Geometry check sheet. Reference: the model listing, model coordinates, mm. Face numbers are marked on the shaded views. A direction names the side the tool comes from. Round coordinates to 2 decimals unless told otherwise and drop trailing zeros. Loops run counter-clockwise (first coordinate to the right, second up) from the corner with the lowest first, then second, coordinate; pieces in that order, holes last. Notation, with made-up numbers: (-39, 15) - (-14, 15) arc R4 cw to (-14, 20) - close; hole circle Ø3 at (64.25, 14). An arc over 180 degrees is marked (long way). Answer as CSV lines item,"result". Start each with the question number.
1) Cross-section at A-A on y = 0. Record the boundary of the cut face in (x, z).
2) Thickness scan on line 1 along Y through (x, z) = (0, -2.15); line 2 along Z through (x, y) = (12.5, -9.5); line 3 along Z through (x, y) = (11, 13). Record the ranges inside material, lowest first.
3) Cross-section at B-B on z = -32.5. Record the boundary of the cut face in (x, y), and give its area (3 significant figures).
4) Cross-section at D-D on y = 4. Record the boundary of the cut face in (x, z).
5) Depth check by flat-ended pin: P1, Ø1.5, axis at x = -3.5, z = -52.5, coming from the -Y side; P2, Ø4, axis at x = 0, y = 15.5, coming from the +Z side; P3, Ø1, axis at y = -14.5, z = -46.5, coming from the -X side; P4, Ø11, axis at x = 2.5, y = -4.5, coming from the +Z side. Enter the tip coordinate at first touch or a pass-through.
6) Access from +Z, -Z, +X, -X, +Y, -Y to the whole of each face (thin tool, end or side, straight path). Record for the marked faces 1, 2 and 3.
7) Cross-section at C-C on x = 6. Record the boundary of the cut face in (y, z), and give its area (3 significant figures).
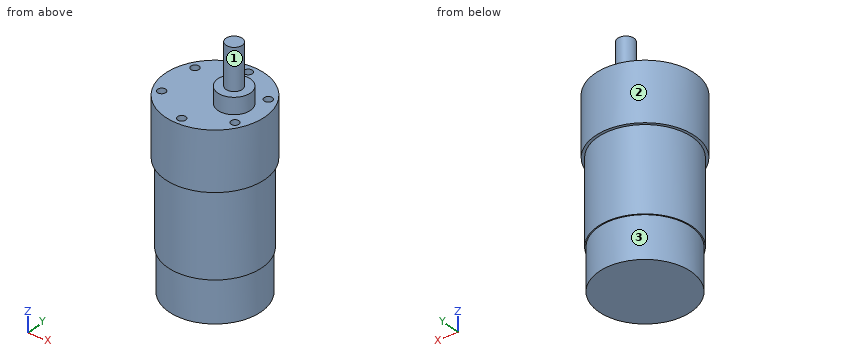
from build123d import *

# Parameters (mm, degrees)
SKETCH_1_R          = 18.4
EXTRUDE_1_DEPTH     = 21.5
SKETCH_1_3_R        = 6
EXTRUDE_2_DEPTH     = 6
SKETCH_1_4_R        = 3
EXTRUDE_3_DEPTH     = 21.2
SKETCH_2_R          = 17.4
EXTRUDE_4_DEPTH     = 30.7
EXTRUDE_START       = 30.7
SKETCH_2_3_R        = 17
EXTRUDE_5_DEPTH     = 15.4
SKETCH_1_5_R        = 1.5
CUT_EXTRUDE_1_DEPTH = 5


with BuildPart() as part:
    # 스케치1 → 보스-돌출1 (new body)
    with BuildSketch(Plane.XY):
        Circle(SKETCH_1_R)
    extrude(amount=-EXTRUDE_1_DEPTH)

    # 스케치1<3> → 보스-돌출2 (add)
    with BuildSketch(Plane.XY):
        with Locations((7, 0)):
            Circle(SKETCH_1_3_R)
    extrude(amount=EXTRUDE_2_DEPTH)

    # 스케치1<4> → 보스-돌출3 (add)
    with BuildSketch(Plane.XY):
        with Locations((7, 0)):
            Circle(SKETCH_1_4_R)
    extrude(amount=EXTRUDE_3_DEPTH)

    # 스케치2 → 보스-돌출4 (add)
    with BuildSketch(Plane(origin=(0, 0, -21.5), x_dir=(-1, 0, 0), z_dir=(0, 0, -1))):
        Circle(SKETCH_2_R)
    extrude(amount=EXTRUDE_4_DEPTH)

    # 스케치2<3> → 보스-돌출5 (add)
    with BuildSketch(Plane(origin=(0, 0, -21.5), x_dir=(-1, 0, 0), z_dir=(0, 0, -1)).offset(EXTRUDE_START)):
        with Locations(Location((0, 0, 0), (0, 0, 180))):
            Circle(SKETCH_2_3_R)
    extrude(amount=EXTRUDE_5_DEPTH)

    # 스케치1<5> → 컷-돌출1 (cut)
    with BuildSketch(Plane.XY):
        with Locations((-13.423393759, -7.75)):
            Circle(SKETCH_1_5_R)
        with Locations((-13.423393759, 7.75)):
            Circle(SKETCH_1_5_R)
        with Locations((0, 15.5)):
            Circle(SKETCH_1_5_R)
        with Locations((13.423393759, 7.75)):
            Circle(SKETCH_1_5_R)
        with Locations((13.423393759, -7.75)):
            Circle(SKETCH_1_5_R)
        with Locations((0, -15.5)):
            Circle(SKETCH_1_5_R)
    extrude(amount=-CUT_EXTRUDE_1_DEPTH, mode=Mode.SUBTRACT)


solid = part.part
Answer block:
1,outline,"(-18.4, -21.5) - (-17.4, -21.5) - (-17.4, -52.2) - (-17, -52.2) - (-17, -67.6) - (17, -67.6) - (17, -52.2) - (17.4, -52.2) - (17.4, -21.5) - (18.4, -21.5) - (18.4, 0) - (13, 0) - (13, 6) - (10, 6) - (10, 21.2) - (4, 21.2) - (4, 6) - (1, 6) - (1, 0) - (-18.4, 0) - close"
2,line 1,"y = -18.4 to -17, -14 to 14, 17 to 18.4"
2,line 2,"z = -67.6 to 0"
2,line 3,"z = -52.2 to 0"
3,outline,"circle Ø34.8 at (0, 0)"
3,area,"951 mm^2"
4,outline,"(-17.96, -21.5) - (-16.93, -21.5) - (-16.93, -52.2) - (-16.52, -52.2) - (-16.52, -67.6) - (16.52, -67.6) - (16.52, -52.2) - (16.93, -52.2) - (16.93, -21.5) - (17.96, -21.5) - (17.96, 0) - (11.47, 0) - (11.47, 6) - (2.53, 6) - (2.53, 0) - (-17.96, 0) - close"
5,P1,"stops at y = -17.17"
5,P2,"stops at z = 0"
5,P3,"stops at x = -10.33"
5,P4,"stops at z = 21.2"
6,face 1,"+Z"
6,face 2,"+Z, -Z"
6,face 3,"-Z"
7,outline,"(-17.39, -21.5) - (-16.33, -21.5) - (-16.33, -52.2) - (-15.91, -52.2) - (-15.91, -67.6) - (15.91, -67.6) - (15.91, -52.2) - (16.33, -52.2) - (16.33, -21.5) - (17.39, -21.5) - (17.39, 0) - (5.92, 0) - (5.92, 6) - (2.83, 6) - (2.83, 21.2) - (-2.83, 21.2) - (-2.83, 6) - (-5.92, 6) - (-5.92, 0) - (-17.39, 0) - close"
7,area,"2,400 mm^2"
